Verification items for this drawing (mm, ordinates from the low corner). A direction names the side the tool comes from. Coordinates: 2 decimals unless noted, no trailing zeros. Write each loop counter-clockwise with the first axis right and the second up, starting at its lowest first coordinate (ties: lowest second). Pieces come first, ordered by that corner, then holes. Notation, with made-up numbers: M 70.25,-36 L 108.25,-36 A26 cw 108.25,-8 Z; hole C 50.25,61.5 d3. An arc over 180 degrees is marked long. Write each question's results on one line, items separated by ' | '.
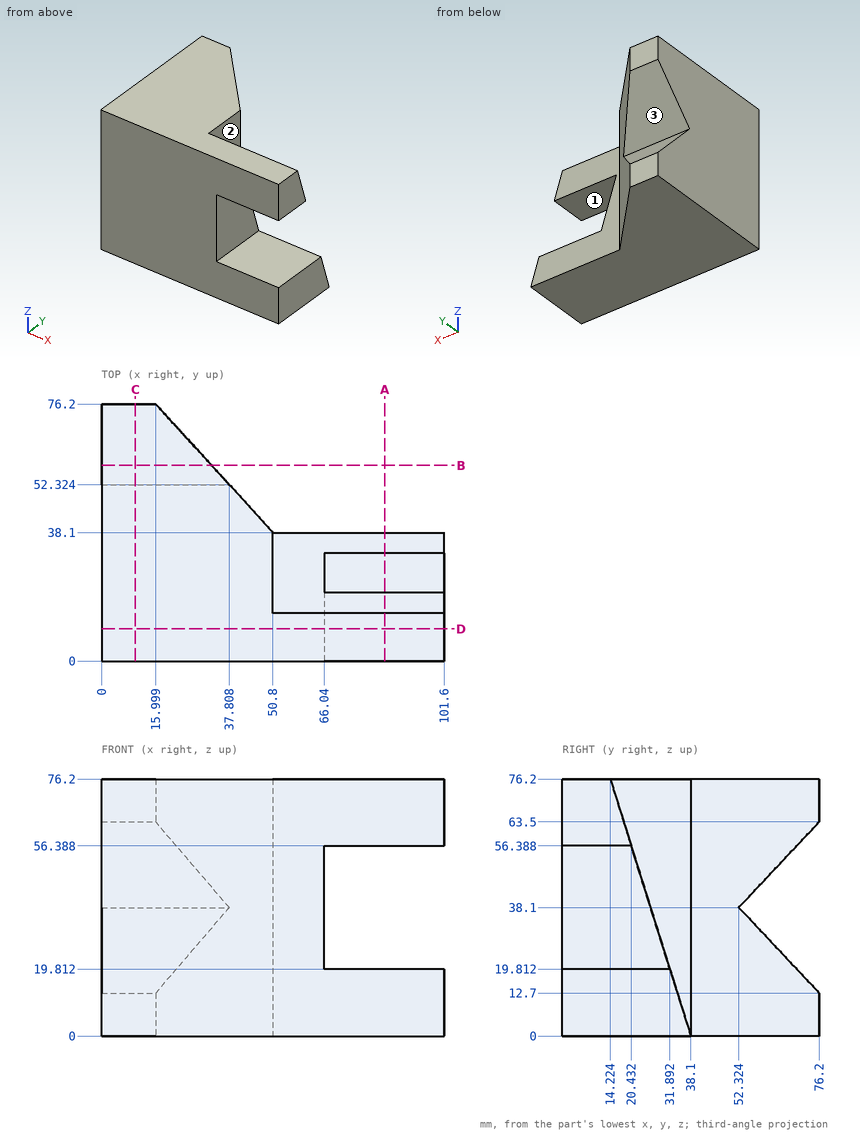
Q1. Sectioned sample at A-A on x = 84. Record the cut outline in (y, z), and give its area (3 significant figures).
Geometry check:
outline: M 0,0 L 38.1,0 L 31.89,19.81 L 0,19.81 Z; M 0,56.39 L 20.43,56.39 L 14.22,76.2 L 0,76.2 Z | area: 1,040 mm2
Q2. Scan lines: probe 1 along X at (y, z) = (32.5, 42.5); probe 2 along X at (y, z) = (4.5, 45.5); probe 3 along Z at (x, y) = (75, 10.5). Record each from-to range of solid material in increasing order.
Geometry check:
probe 1: x = 0 to 50.8 | probe 2: x = 0 to 66.04 | probe 3: z = 0 to 19.81, 56.39 to 76.2
Q3. Sectioned sample at B-B on y = 58. Record the cut outline in (x, z), and give its area (3 significant figures).
Geometry check:
outline: M 0,0 L 32.62,0 L 32.62,32.06 L 0,32.06 Z; M 0,44.14 L 32.62,44.14 L 32.62,76.2 L 0,76.2 Z | area: 2,090 mm2
Q4. Sectioned sample at D-D on y = 9.5. Record the cut outline in (x, z), and give its area (3 significant figures).
Geometry check:
outline: M 0,0 L 101.6,0 L 101.6,19.81 L 66.04,19.81 L 66.04,56.39 L 101.6,56.39 L 101.6,76.2 L 0,76.2 Z | area: 6,440 mm2
Q5. Access from +Z, -Z, +X, -X, +Y, -Y to the whole of each face (thin tool, end or side, straight path). Record for the marked faces 1, 2 and 3.
Geometry check:
face 1: +X, +Y, -Y | face 2: +Z, +X, +Y | face 3: +X, -X, +Y
Q6. Sectioned sample at C-C on x = 10. Record the cut outline in (y, z).
Geometry check:
outline: M 0,0 L 76.2,0 L 76.2,12.7 L 52.32,38.1 L 76.2,63.5 L 76.2,76.2 L 0,76.2 Z
Q7. Depth check by flat-ended pin: P1, Ø5, axis at y = 46.5, z = 44, coming from the +X side; P2, Ø9.5, axis at x = 82.5, y = 18, coming from the +Z side; P3, Ø19, axis at y = 30.5, z = 35.5, coming from the +X side. Enter the tip coordinate at first touch or a pass-through.
Geometry check:
P1: stops at x = 45.41 | P2: stops at z = 76.2 | P3: stops at x = 66.04
